Can you work these out from the model? Positions are in its coordinate system, mm. A direction names the side the tool comes from. Coordinates: 2 decimals unless noted, no trailing zeros. Order: outer loops, then holes, each group sorted by start corner. A loop starts at its lowest first (then second) coordinate and runs counter-clockwise, first axis right, second up. Notation, with made-up numbers: M 20,59.25 L 71,59.25 A25 cw 71,89.25 Z; hole C 2,82 d1. An arc over 180 degrees is marked long. Answer as a JSON object with one key per item and string values.
from build123d import *

# Parameters (mm, degrees)
BOSS_EXTRUDE1_DEPTH = 63.5
CUT_EXTRUDE1_DEPTH  = 92.510528356
SKETCH4_R           = 2.54
CUT_EXTRUDE2_DEPTH  = 92.510528356


with BuildPart() as part:
    # Sketch1 → Boss-Extrude1 (new body)
    with BuildSketch(Plane.XY):
        Polygon((0, 0), (30.48, 0), (30.48, -12.7), (32.512, -12.7), (32.512, 2.032), (2.032, 2.032), (2.032, 58.42), (0, 58.42), align=None)
    extrude(amount=-BOSS_EXTRUDE1_DEPTH)

    # Sketch2 → Cut-Extrude1 (cut, through all)
    with BuildSketch(Plane(origin=(2.032, 0, 0), x_dir=(0, 0, -1), z_dir=(1, 0, 0))):
        Polygon((31.75, 43.18), (36.83, 43.18), (36.83, 33.02), (26.67, 33.02), (26.67, 43.18), align=None)
    extrude(amount=-CUT_EXTRUDE1_DEPTH, mode=Mode.SUBTRACT)

    # Sketch4 → Cut-Extrude2 (cut, through all)
    with BuildSketch(Plane.ZY.offset(-30.48)):
        with Locations((-52.07, -6.35)):
            Circle(SKETCH4_R)
        with Locations(Location((-11.43, -6.35, 0), (0, 0, 180))):
            Circle(SKETCH4_R)
    extrude(amount=-CUT_EXTRUDE2_DEPTH, mode=Mode.SUBTRACT)


solid = part.part
Item 1: I want a section at C-C, the plane y = -6.35. Write out the boundary of the cut face in (x, z), plus the area to 3 significant figures.
Answers follow:
{"outline": "M 30.48,-63.5 L 32.51,-63.5 L 32.51,-54.61 L 30.48,-54.61 Z; M 30.48,-49.53 L 32.51,-49.53 L 32.51,-13.97 L 30.48,-13.97 Z; M 30.48,-8.89 L 32.51,-8.89 L 32.51,0 L 30.48,0 Z", "area": "108 mm^2"}
Item 2: I'm going to push flat-ended pins straight in: pin 1 (15 mm diameter, centred on x = 17.5, z = -21.5, fed in from +Y); pin 2 (2 mm diameter, centred on x = 1.5, z = -32, fed in from -Y); pin 3 (6 mm diameter, centred on y = -6.35, z = -52.07, fed in from +X); pin 4 (6.5 mm diameter, centred on y = -3.5, z = -39.5, fed in from -X). Where does each tip first touch, or does it pass through?
Answers follow:
{"pin 1": "stops at y = 2.03", "pin 2": "stops at y = 0", "pin 3": "stops at x = 32.51", "pin 4": "stops at x = 30.48"}
Item 3: Which directions (+Z, -Z, +X, -X, +Y, -Y) give clear straight access to the entire face, cutting with the end or side of a thin tool? Please do faces 4 (the flat face through (1, 38, -36.83)), 5 (the flat face through (2.032, 30, -31)), 6 (the flat face through (30.48, -6, -31)).
Answers follow:
{"face 4": "+X, -X", "face 5": "+Z, -Z, +X, +Y", "face 6": "+Z, -Z, -X, -Y"}
Item 4: I want a section at D-D, the plane z = -11.43. Write out the boundary of the cut face in (x, y).
Answers follow:
{"outline": "M 0,0 L 30.48,0 L 30.48,-3.81 L 32.51,-3.81 L 32.51,2.03 L 2.03,2.03 L 2.03,58.42 L 0,58.42 Z; M 30.48,-12.7 L 32.51,-12.7 L 32.51,-8.89 L 30.48,-8.89 Z"}
Item 5: I want a section at B-B, the plane y = 34.5. Write out the boundary of the cut face in (x, z).
Answers follow:
{"outline": "M 0,-63.5 L 2.03,-63.5 L 2.03,-36.83 L 0,-36.83 Z; M 0,-26.67 L 2.03,-26.67 L 2.03,0 L 0,0 Z"}
Item 6: I want a section at A-A, the plane z = -35.5. Write out the boundary of the cut face in (x, y).
Answers follow:
{"outline": "M 0,0 L 30.48,0 L 30.48,-12.7 L 32.51,-12.7 L 32.51,2.03 L 2.03,2.03 L 2.03,33.02 L 0,33.02 Z; M 0,43.18 L 2.03,43.18 L 2.03,58.42 L 0,58.42 Z"}
Item 7: Please list where these lines run through material, in increasing order: line 1 (Y direction, x = 31.15, z = -52.07); line 2 (X direction, y = 27.5, z = -41.5); line 3 (Z direction, x = 2, y = 43).
Answers follow:
{"line 1": "y = -12.7 to -8.89, -3.81 to 2.03", "line 2": "x = 0 to 2.03", "line 3": "z = -63.5 to -36.83, -26.67 to 0"}
Item 8: If we mould it in two halves opening along Z, with no side actions, what happens to faces 1 (the flat face through (1.7, 15.1, 0)), 2 (the flat face through (17, 2.032, -31)), 3 (the flat face through (1, 33.02, -32))? For each: pulls with the +Z half, pulls with the -Z half, needs draft (parallel to the pull), parting line crosses it, or undercut.
Answers follow:
{"face 1": "pulls with the +Z half", "face 2": "needs draft", "face 3": "undercut"}
